CAD build for the part. Positions are in the model's coordinates, mm. A direction names the side the tool comes from. Coordinates: 2 decimals unless noted, no trailing zeros. Loops run counter-clockwise (first coordinate to the right, second up) from the corner with the lowest first, then second, coordinate; pieces in that order, holes last. Notation, with made-up numbers: (3, 40.25) -> (47, 40.25) arc R10 ccw to (47, 52.25) -> close; hole circle Ø4 at (86, -28.5). An arc over 180 degrees is marked (long way). Return JSON: item names as keys, results as strings. Group by question number.
(1) Saw through at D-D on x = 96.5. Write the cut outline in (y, z), then the cut area to 3 significant figures.
(2) Probe L1, parallel to X at y = 147, z = -335; L2, parallel to X at y = 3, z = -397; L3, parallel to Z at x = 361.95, y = 2.75 (3 decimals). List the from-to ranges inside material, lowest first.
(3) Saw through at C-C on z = -437. Write the cut outline in (x, y), then the cut area to 3 significant figures.
(4) Saw through at B-B on z = -365.76. Write the cut outline in (x, y).
(5) Saw through at A-A on y = 90.5. Write the cut outline in (x, z).
(6) Mould opens along Z. For faces 1 (the face through (105, 3, -284.48)), 2 (the face through (377.87, 11.49, -372.36)), 3 (the face through (3.13, 11.49, -359.16)), 4 (the face through (6.35, 103, -381)) say: pulls with the +Z half, pulls with the -Z half, needs draft (parallel to the pull), parting line crosses it, or undercut.
(7) Tool access for faces 5 (the face through (193, 0, -356)), 6 (the face through (147, 5, -429.26)), 7 (the face through (374.65, 106, -381)): list every direction of +Z, -Z, +X, -X, +Y, -Y with a clear straight run to the whole face (end or side of a thin tool).
(8) Flat gauge pins, fed straight in: pin 1 Ø4 at (y, z) = (193.68, -302.44) entering from -X; pin 2 Ø10 at (x, z) = (304.8, -309.88) entering from +Y; pin 3 Ø3 at (y, z) = (106.8, -301.4) entering from +X; pin 4 Ø1.5 at (x, z) = (165, -416.5) entering from +Y. Where does each tip first touch, or does it go through?
```python
from build123d import *

# Parameters (mm, degrees)
SKETCH1_W            = 381
SKETCH1_H            = 429.26
BOSS_EXTRUDE1_DEPTH  = 6.35
SKETCH2_W            = 254
SKETCH2_H            = 203.2
CUT_EXTRUDE1_DEPTH   = 6.35
SKETCH3_W            = 381
SKETCH3_H            = 73.66
CUT_EXTRUDE2_DEPTH   = 6.35
SKETCH4_W            = 254
SKETCH4_H            = 6.35
CUT_EXTRUDE3_DEPTH   = 73.66
SKETCH6_W            = 6.35
SKETCH6_H            = 195.58
BOSS_EXTRUDE2_DEPTH  = 171.45
SKETCH7_W            = 6.35
SKETCH7_H            = 195.58
BOSS_EXTRUDE3_DEPTH  = 158.75
SKETCH8_W            = 6.35
SKETCH8_H            = 165.1
BOSS_EXTRUDE4_DEPTH  = 50.8
SKETCH9_W            = 6.35
SKETCH9_H            = 158.75
CUT_EXTRUDE4_DEPTH   = 50.8
SKETCH10_W           = 6.899940386
SKETCH10_H           = 177.8
BOSS_EXTRUDE5_DEPTH  = 50.8
SKETCH11_W           = 6.35
SKETCH11_H           = 171.45
CUT_EXTRUDE5_DEPTH   = 50.8
SKETCH13_W           = 0.549940386
SKETCH13_H           = 171.45
CUT_EXTRUDE6_DEPTH   = 50.8
SKETCH14_W           = 6.899940386
SKETCH14_H           = 177.8
CUT_EXTRUDE7_DEPTH   = 50.8
SKETCH15_W           = 6.35
SKETCH15_H           = 165.1
CUT_EXTRUDE8_DEPTH   = 50.8
SKETCH16_W           = 6.35
SKETCH16_H           = 144.78
BOSS_EXTRUDE6_DEPTH  = 25.4
SKETCH17_W           = 6.35
SKETCH17_H           = 144.78
BOSS_EXTRUDE7_DEPTH  = 19.05
SKETCH19_W           = 6.35
SKETCH19_H           = 139.7
BOSS_EXTRUDE8_DEPTH  = 50.8
SKETCH20_W           = 6.35
SKETCH20_H           = 195.58
BOSS_EXTRUDE9_DEPTH  = 31.75
SKETCH21_W           = 6.35
SKETCH21_H           = 139.7
BOSS_EXTRUDE10_DEPTH = 50.8
SKETCH22_W           = 6.35
SKETCH22_H           = 195.58
BOSS_EXTRUDE11_DEPTH = 50.8
SKETCH23_W           = 6.35
SKETCH23_H           = 50.8
BOSS_EXTRUDE12_DEPTH = 12.7
SKETCH24_W           = 6.35
SKETCH24_H           = 195.58
BOSS_EXTRUDE13_DEPTH = 12.7
SKETCH26_W           = 381
SKETCH26_H           = 210.82
CUT_EXTRUDE9_DEPTH   = 12.7
SKETCH27_R           = 7.14375
CUT_EXTRUDE12_DEPTH  = 8.89
SKETCH29_R           = 7.14375
CUT_EXTRUDE13_DEPTH  = 8.89
SKETCH31_R           = 3.175
CUT_EXTRUDE14_DEPTH  = 12.7
SKETCH36_R           = 1.905
CUT_EXTRUDE17_DEPTH  = 12.7
SKETCH37_R           = 2.667
CUT_EXTRUDE18_DEPTH  = 17.78
SKETCH38_R           = 3.175
CUT_EXTRUDE19_DEPTH  = 17.78
SKETCH39_R           = 3.175
CUT_EXTRUDE20_DEPTH  = 17.78
SKETCH41_R           = 3.175
CUT_EXTRUDE21_DEPTH  = 15.24
SKETCH42_R           = 3.302
CUT_EXTRUDE22_DEPTH  = 12.7
SKETCH43_R           = 3.302
SKETCH43_R_2         = 3.175
SKETCH43_R_3         = 3.175000007
BOSS_EXTRUDE14_DEPTH = 6.35


with BuildPart() as part:
    # Sketch1 → Boss-Extrude1 (new body)
    with BuildSketch(Plane(origin=(0, 0, 0), x_dir=(1, 0, 0), z_dir=(0, 1, 0))):
        with Locations((190.5, 214.63)):
            Rectangle(SKETCH1_W, SKETCH1_H)
    extrude(amount=BOSS_EXTRUDE1_DEPTH)

    # Sketch2 → Cut-Extrude1 (cut)
    with BuildSketch(Plane(origin=(0, 6.35, 0), x_dir=(1, 0, 0), z_dir=(0, 1, 0))):
        with Locations((190.5, 101.6)):
            Rectangle(SKETCH2_W, SKETCH2_H)
    extrude(amount=-CUT_EXTRUDE1_DEPTH, mode=Mode.SUBTRACT)

    # Sketch3 → Cut-Extrude2 (cut)
    with BuildSketch(Plane(origin=(0, 6.35, 0), x_dir=(1, 0, 0), z_dir=(0, 1, 0))):
        with Locations((190.5, 36.83)):
            Rectangle(SKETCH3_W, SKETCH3_H)
    extrude(amount=-CUT_EXTRUDE2_DEPTH, mode=Mode.SUBTRACT)

    # Sketch4 → Cut-Extrude3 (cut)
    with BuildSketch(Plane.XY.offset(-203.2)):
        with Locations((190.5, 3.175)):
            Rectangle(SKETCH4_W, SKETCH4_H)
    extrude(amount=-CUT_EXTRUDE3_DEPTH, mode=Mode.SUBTRACT)

    # Sketch6 → Boss-Extrude2 (add)
    with BuildSketch(Plane(origin=(0, 6.35, 0), x_dir=(1, 0, 0), z_dir=(0, 1, 0))):
        with Locations((377.825, 331.47)):
            Rectangle(SKETCH6_W, SKETCH6_H)
    extrude(amount=BOSS_EXTRUDE2_DEPTH)

    # Sketch7 → Boss-Extrude3 (add)
    with BuildSketch(Plane(origin=(0, 6.35, 0), x_dir=(1, 0, 0), z_dir=(0, 1, 0))):
        with Locations((3.175, 331.47)):
            Rectangle(SKETCH7_W, SKETCH7_H)
    extrude(amount=BOSS_EXTRUDE3_DEPTH)

    # Sketch8 → Boss-Extrude4 (add)
    with BuildSketch(Plane(origin=(0, 0, -429.26), x_dir=(-1, 0, 0), z_dir=(0, 0, -1))):
        with Locations((-3.175, 82.55)):
            Rectangle(SKETCH8_W, SKETCH8_H)
    extrude(amount=BOSS_EXTRUDE4_DEPTH)

    # Sketch9 → Cut-Extrude4 (cut)
    with BuildSketch(Plane.XY.offset(-233.68)):
        with Locations((3.175, 85.725)):
            Rectangle(SKETCH9_W, SKETCH9_H)
    extrude(amount=-CUT_EXTRUDE4_DEPTH, mode=Mode.SUBTRACT)

    # Sketch10 → Boss-Extrude5 (add)
    with BuildSketch(Plane(origin=(0, 0, -429.26), x_dir=(-1, 0, 0), z_dir=(0, 0, -1))):
        with Locations((-377.550029807, 88.9)):
            Rectangle(SKETCH10_W, SKETCH10_H)
    extrude(amount=BOSS_EXTRUDE5_DEPTH)

    # Sketch11 → Cut-Extrude5 (cut)
    with BuildSketch(Plane.XY.offset(-233.68)):
        with Locations((377.825, 92.075)):
            Rectangle(SKETCH11_W, SKETCH11_H)
    extrude(amount=-CUT_EXTRUDE5_DEPTH, mode=Mode.SUBTRACT)

    # Sketch13 → Cut-Extrude6 (cut)
    with BuildSketch(Plane.XY.offset(-429.26)):
        with Locations((374.375029807, 92.075)):
            Rectangle(SKETCH13_W, SKETCH13_H)
    extrude(amount=-CUT_EXTRUDE6_DEPTH, mode=Mode.SUBTRACT)

    # Sketch14 → Cut-Extrude7 (cut)
    with BuildSketch(Plane(origin=(0, 0, -480.06), x_dir=(-1, 0, 0), z_dir=(0, 0, -1))):
        with Locations((-377.550029807, 88.9)):
            Rectangle(SKETCH14_W, SKETCH14_H)
    extrude(amount=-CUT_EXTRUDE7_DEPTH, mode=Mode.SUBTRACT)

    # Sketch15 → Cut-Extrude8 (cut)
    with BuildSketch(Plane(origin=(0, 0, -480.06), x_dir=(-1, 0, 0), z_dir=(0, 0, -1))):
        with Locations((-3.175, 82.55)):
            Rectangle(SKETCH15_W, SKETCH15_H)
    extrude(amount=-CUT_EXTRUDE8_DEPTH, mode=Mode.SUBTRACT)

    # Sketch16 → Boss-Extrude6 (add)
    with BuildSketch(Plane(origin=(0, 177.8, 0), x_dir=(1, 0, 0), z_dir=(0, 1, 0))):
        with Locations((377.825, 356.87)):
            Rectangle(SKETCH16_W, SKETCH16_H)
    extrude(amount=BOSS_EXTRUDE6_DEPTH)

    # Sketch17 → Boss-Extrude7 (add)
    with BuildSketch(Plane(origin=(0, 165.1, 0), x_dir=(1, 0, 0), z_dir=(0, 1, 0))):
        with Locations((3.175, 356.87)):
            Rectangle(SKETCH17_W, SKETCH17_H)
    extrude(amount=-BOSS_EXTRUDE7_DEPTH)

    # Sketch19 → Boss-Extrude8 (add)
    with BuildSketch(Plane(origin=(0, 0, -429.26), x_dir=(-1, 0, 0), z_dir=(0, 0, -1))):
        with Locations((-3.175, 120.65)):
            Rectangle(SKETCH19_W, SKETCH19_H)
    extrude(amount=BOSS_EXTRUDE8_DEPTH)

    # Sketch20 → Boss-Extrude9 (add)
    with BuildSketch(Plane(origin=(0, 190.5, 0), x_dir=(1, 0, 0), z_dir=(0, 1, 0))):
        with Locations((3.175, 382.27)):
            Rectangle(SKETCH20_W, SKETCH20_H)
    extrude(amount=-BOSS_EXTRUDE9_DEPTH)

    # Sketch21 → Boss-Extrude10 (add)
    with BuildSketch(Plane(origin=(0, 0, -429.26), x_dir=(-1, 0, 0), z_dir=(0, 0, -1))):
        with Locations((-377.825, 133.35)):
            Rectangle(SKETCH21_W, SKETCH21_H)
    extrude(amount=BOSS_EXTRUDE10_DEPTH)

    # Sketch22 → Boss-Extrude11 (add)
    with BuildSketch(Plane(origin=(0, 203.2, 0), x_dir=(1, 0, 0), z_dir=(0, 1, 0))):
        with Locations((377.825, 382.27)):
            Rectangle(SKETCH22_W, SKETCH22_H)
    extrude(amount=-BOSS_EXTRUDE11_DEPTH)

    # Sketch23 → Boss-Extrude12 (add)
    with BuildSketch(Plane.XZ.offset(-63.5)):
        with Locations((377.825, -454.66)):
            Rectangle(SKETCH23_W, SKETCH23_H)
    extrude(amount=BOSS_EXTRUDE12_DEPTH)

    # Sketch24 → Boss-Extrude13 (add)
    with BuildSketch(Plane(origin=(0, 190.5, 0), x_dir=(1, 0, 0), z_dir=(0, 1, 0))):
        with Locations((3.175, 382.27)):
            Rectangle(SKETCH24_W, SKETCH24_H)
    extrude(amount=BOSS_EXTRUDE13_DEPTH)

    # Sketch26 → Cut-Extrude9 (cut)
    with BuildSketch(Plane(origin=(0, 6.35, 0), x_dir=(1, 0, 0), z_dir=(0, 1, 0))):
        with Locations((190.5, 179.07)):
            Rectangle(SKETCH26_W, SKETCH26_H)
    extrude(amount=-CUT_EXTRUDE9_DEPTH, mode=Mode.SUBTRACT)

    # Sketch27 → Cut-Extrude12 (cut)
    with BuildSketch(Plane.ZY):
        with Locations((-365.76, 14.224)):
            Circle(SKETCH27_R)
    extrude(amount=-CUT_EXTRUDE12_DEPTH, mode=Mode.SUBTRACT)

    # Sketch29 → Cut-Extrude13 (cut)
    with BuildSketch(Plane(origin=(381, 0, 0), x_dir=(0, 0, -1), z_dir=(1, 0, 0))):
        with Locations((365.76, 14.224)):
            Circle(SKETCH29_R)
    extrude(amount=-CUT_EXTRUDE13_DEPTH, mode=Mode.SUBTRACT)

    # Sketch31 → Cut-Extrude14 (cut)
    with BuildSketch(Plane(origin=(0, 6.35, 0), x_dir=(1, 0, 0), z_dir=(0, 1, 0))):
        with Locations((368.3, 416.56)):
            Circle(SKETCH31_R)
        with Locations((304.8, 416.56)):
            Circle(SKETCH31_R)
        with Locations((12.7, 416.56)):
            Circle(SKETCH31_R)
        with Locations((76.2, 416.56)):
            Circle(SKETCH31_R)
    extrude(amount=-CUT_EXTRUDE14_DEPTH, mode=Mode.SUBTRACT)

    # Sketch36 → Cut-Extrude17 (cut)
    with BuildSketch(Plane(origin=(381, 0, 0), x_dir=(0, 0, -1), z_dir=(1, 0, 0))):
        with Locations((344.451335942, 154.548846533)):
            Circle(SKETCH36_R)
        with Locations((301.398335942, 154.5512)):
            Circle(SKETCH36_R)
        with Locations((344.451335942, 106.7992)):
            Circle(SKETCH36_R)
        with Locations((301.398335942, 106.7992)):
            Circle(SKETCH36_R)
    extrude(amount=-CUT_EXTRUDE17_DEPTH, mode=Mode.SUBTRACT)

    # Sketch37 → Cut-Extrude18 (cut)
    with BuildSketch(Plane(origin=(0, 6.35, 0), x_dir=(1, 0, 0), z_dir=(0, 1, 0))):
        with Locations((63.5, 397.51)):
            Circle(SKETCH37_R)
        with Locations((63.5, 293.116)):
            Circle(SKETCH37_R)
        with Locations((245.7704, 293.116)):
            Circle(SKETCH37_R)
        with Locations((245.7704, 397.51)):
            Circle(SKETCH37_R)
    extrude(amount=-CUT_EXTRUDE18_DEPTH, mode=Mode.SUBTRACT)

    # Sketch38 → Cut-Extrude19 (cut)
    with BuildSketch(Plane(origin=(0, 6.35, 0), x_dir=(1, 0, 0), z_dir=(0, 1, 0))):
        with Locations((304.8, 309.88)):
            Circle(SKETCH38_R)
        with Locations((361.95, 337.82)):
            Circle(SKETCH38_R)
    extrude(amount=-CUT_EXTRUDE19_DEPTH, mode=Mode.SUBTRACT)

    # Sketch39 → Cut-Extrude20 (cut)
    with BuildSketch(Plane.ZY):
        with Locations((-454.84383327, 190.5)):
            Circle(SKETCH39_R)
        with Locations((-302.443833262, 193.675)):
            Circle(SKETCH39_R)
    extrude(amount=-CUT_EXTRUDE20_DEPTH, mode=Mode.SUBTRACT)

    # Sketch41 → Cut-Extrude21 (cut)
    with BuildSketch(Plane.ZY):
        with Locations((-424.2308, 149.9108)):
            Circle(SKETCH41_R)
        with Locations((-290.8808, 48.387)):
            Circle(SKETCH41_R)
        with Locations((-290.8808, 149.9108)):
            Circle(SKETCH41_R)
    extrude(amount=-CUT_EXTRUDE21_DEPTH, mode=Mode.SUBTRACT)

    # Sketch42 → Cut-Extrude22 (cut)
    with BuildSketch(Plane(origin=(381, 0, 0), x_dir=(0, 0, -1), z_dir=(1, 0, 0))):
        with Locations((454.843833262, 190.5)):
            Circle(SKETCH42_R)
        with Locations((302.443833262, 193.675)):
            Circle(SKETCH42_R)
    extrude(amount=-CUT_EXTRUDE22_DEPTH, mode=Mode.SUBTRACT)

    # Sketch43 → Boss-Extrude14 (add)
    with BuildSketch(Plane(origin=(381, 0, 0), x_dir=(0, 0, -1), z_dir=(1, 0, 0))):
        with Locations((302.443833262, 193.675)):
            Circle(SKETCH43_R)
        with Locations((302.443833262, 193.675)):
            Circle(SKETCH43_R_2, mode=Mode.SUBTRACT)
        with Locations((454.843833262, 190.5)):
            Circle(SKETCH43_R)
        with Locations((454.843833262, 190.5)):
            Circle(SKETCH43_R_3, mode=Mode.SUBTRACT)
    extrude(amount=-BOSS_EXTRUDE14_DEPTH)


solid = part.part
```
Geometry results:
{
 "1": {"outline": "(0, -429.26) -> (6.35, -429.26) -> (6.35, -284.48) -> (0, -284.48) -> close", "area": "919 mm²"},
 "2": {"L1": "0 to 6.35, 374.65 to 381", "L2": "0 to 60.88, 66.12 to 243.15, 248.39 to 381", "L3": "-429.26 to -340.995, -334.645 to -284.48"},
 "3": {"outline": "(0, 50.8) -> (6.35, 50.8) -> (6.35, 203.2) -> (0, 203.2) -> close; (374.65, 50.8) -> (381, 50.8) -> (381, 203.2) -> (374.65, 203.2) -> close", "area": "1,940 mm²"},
 "4": {"outline": "(0, 0) -> (381, 0) -> (381, 7.08) -> (374.65, 7.08) -> (374.65, 6.35) -> (6.35, 6.35) -> (6.35, 7.08) -> (0, 7.08) -> close; (0, 21.37) -> (6.35, 21.37) -> (6.35, 203.2) -> (0, 203.2) -> close; (374.65, 21.37) -> (381, 21.37) -> (381, 203.2) -> (374.65, 203.2) -> close"},
 "5": {"outline": "(0, -480.06) -> (6.35, -480.06) -> (6.35, -284.48) -> (0, -284.48) -> close; (374.65, -480.06) -> (381, -480.06) -> (381, -284.48) -> (374.65, -284.48) -> close"},
 "6": {"face 1": "pulls with the +Z half", "face 2": "undercut", "face 3": "undercut", "face 4": "needs draft"},
 "7": {"face 5": "+Z, -Z, +X, -X, -Y", "face 6": "-Z, +X, -X, -Y", "face 7": "+Z, -Z, +Y"},
 "8": {"pin 1": "through", "pin 2": "y = 6.35", "pin 3": "x = 6.35", "pin 4": "y = 6.35"}
}
